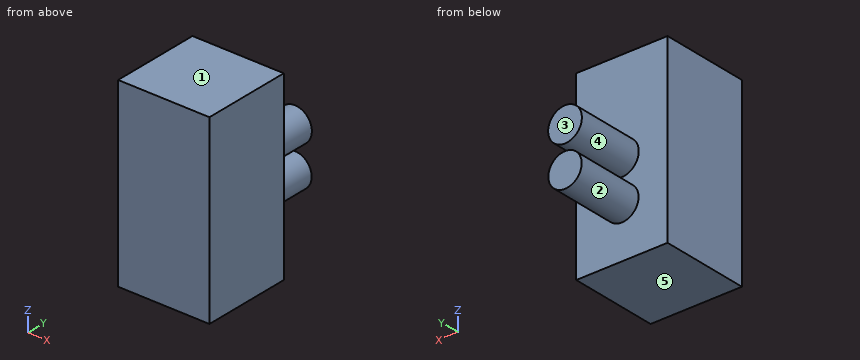
from build123d import *

# Parameters (mm, degrees)
F0_W     = 25.4
F0_H     = 50.8
F1_DEPTH = 24.892
F2_R     = 4.6961896277
F2_R_2   = 4.6352376904
F3_DEPTH = 19.05


# Not quite as in the source:
# - a feature names something its author has since deleted; it is built from what else it names


with BuildPart() as f1:
    # F0 (on Front) → F1 (new body)
    with BuildSketch(Plane.XZ):
        Rectangle(F0_W, F0_H)
    extrude(amount=F1_DEPTH)

    # F2 (on Front) → F3 (join)
    with BuildSketch(Plane.XZ):
        Circle(F2_R)
        with Locations((0, -11.2072117627)):
            Circle(F2_R_2)
    extrude(amount=-F3_DEPTH)


solid = f1.part
Here's how the part is built. I have some questions about the finished solid (model axes, mm). Face numbers are marked on the shaded views. A direction names the side the tool comes from. Round coordinates to 2 decimals unless told otherwise and drop trailing zeros. Write each loop counter-clockwise with the first axis right and the second up, starting at its lowest first coordinate (ties: lowest second). Pieces come first, ordered by that corner, then holes.
1. If we mould it in two halves opening along Z, with no side actions, what happens to the marked faces 1, 2 and 3? For each: released by +Z, released by -Z, zero draft, split by the parting line, or undercut.
2. Suppose I cut it at B-B (z = 0). List the corners of the cut face in (x, y) for me.
3. I need wall thicknesses on L1, parallel to Y at x = 10.75, z = -3; L2, parallel to Z at x = 1.5, y = 14; L3, parallel to X at y = 12, z = -8. Which ranges of each line are inside material? Lowest first, please.
4. Suppose I cut it at A-A (x = 0). List the corners of the cut face in (y, z) for me.
5. For the marked faces 4 and 5, which set-ups out of +Z, -Z, +X, -X, +Y, -Y let a thin tool reach every point of the face, with its end or its side?
6. Will these pins go through, and if not, where does the flat tip stop? pin 1 Ø10 at (x, z) = (8, 10) entering from +Y; pin 2 Ø6 at (x, y) = (6, 14.5) entering from -Z; pin 3 Ø7.5 at (x, z) = (3, -6) entering from +Y.
7. Suppose I cut it at D-D (x = 4). List the corners of the cut face in (y, z) for me, and give its area (3 significant figures).
8. Suppose I cut it at C-C (y = 2.5). List the corners of the cut face in (x, z) for me.
Answer sheet:
1. face 1: released by +Z
1. face 2: undercut
1. face 3: zero draft
2. outline: (-12.7, -24.89) - (12.7, -24.89) - (12.7, 0) - (4.7, 0) - (4.7, 19.05) - (-4.7, 19.05) - (-4.7, 0) - (-12.7, 0) - close
3. L1: y = -24.89 to 0
3. L2: z = -15.59 to -6.82, -4.45 to 4.45
3. L3: x = -3.35 to 3.35
4. outline: (-24.89, -25.4) - (0, -25.4) - (0, -15.84) - (19.05, -15.84) - (19.05, -6.57) - (0, -6.57) - (0, -4.7) - (19.05, -4.7) - (19.05, 4.7) - (0, 4.7) - (0, 25.4) - (-24.89, 25.4) - close
5. face 4: +Y
5. face 5: -Z, +X, -X, +Y, -Y
6. pin 1: stops at y = 0
6. pin 2: stops at z = -14.74
6. pin 3: stops at y = 19.05
7. outline: (-24.89, -25.4) - (0, -25.4) - (0, -13.55) - (19.05, -13.55) - (19.05, -8.87) - (0, -8.87) - (0, -2.46) - (19.05, -2.46) - (19.05, 2.46) - (0, 2.46) - (0, 25.4) - (-24.89, 25.4) - close
7. area: 1,450 mm2
8. outline: circle Ø9.39 at (0, 0); circle Ø9.27 at (0, -11.21)
